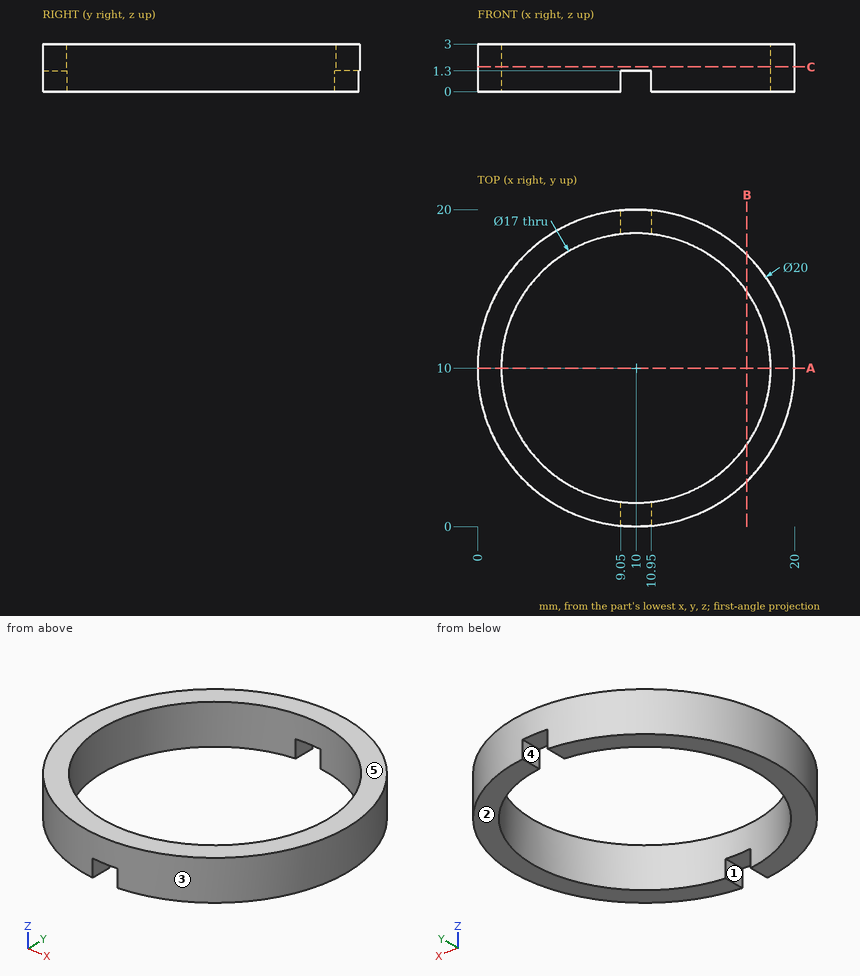
Part print with two shaded views. Sizes in mm from the minimum x, y, z corner. A direction names the side the tool comes from. Coordinates: 2 decimals unless noted, no trailing zeros. Order: outer loops, then holes, each group sorted by start corner. A loop starts at its lowest first (then second) coordinate and runs counter-clockwise, first axis right, second up. Notation, with made-up numbers: (69, 45) - (106, 45) arc R34 ccw to (106, 81) - close; hole circle Ø1 at (87.25, -31). An arc over 180 degrees is marked (long way). Answer in a Markdown table with one row per item.
1. Drill centre lines: L1, parallel to X at y = 10, z = 2; L2, parallel to X at y = 2.5, z = 2.85. Where is each one in solid material? Low to high. Write a range as from..to.
Answer:
| item | result |
|---|---|
| L1 | 0..1.5, 18.5..20 |
| L2 | 3.39..6, 14..16.61 |
2. Slice it at A-A, the plane y = 10. List the corners of the cut face in (x, z), then the cut area to 3 significant figures.
Answer:
| item | result |
|---|---|
| outline | (0, 0) - (1.5, 0) - (1.5, 3) - (0, 3) - close; (18.5, 0) - (20, 0) - (20, 3) - (18.5, 3) - close |
| area | 9.00 mm² |
3. Pull direction X, two halves, no side cores. Call the marked faces 3, 4 and 5: +X half, -X half, draft (parallel to the pull), parting line (faces both ways), or undercut.
Answer:
| item | result |
|---|---|
| face 3 | parting line |
| face 4 | undercut |
| face 5 | draft |
4. Slice it at B-B, the plane x = 17. List the corners of the cut face in (y, z).
Answer:
| item | result |
|---|---|
| outline | (2.86, 0) - (5.18, 0) - (5.18, 3) - (2.86, 3) - close; (14.82, 0) - (17.14, 0) - (17.14, 3) - (14.82, 3) - close |
5. 3-axis set-ups, long thin cutter, end or side, ignore diameter. For the marked faces 1 and 2: which of +Z, -Z, +X, -X, +Y, -Y reach the whole face in a straight line?
Answer:
| item | result |
|---|---|
| face 1 | -Z, +Y, -Y |
| face 2 | -Z, +X, -X, +Y, -Y |
6. Flat gauge pins, fed straight in: P1, Ø0.5, axis at x = 9.5, y = 19.5, coming from the -Z side; P2, Ø1.4, axis at y = 1, z = 1, coming from the -X side; P3, Ø1, axis at y = 1, z = 0.5, coming from the +X side. Where does each tip first touch, or does it go through?
Answer:
| item | result |
|---|---|
| P1 | z = 1.3 |
| P2 | x = 4.42 |
| P3 | x = 15.27 |
7. Slice it at C-C, the plane z = 1.55. List the corners of the cut face in (x, y).
Answer:
| item | result |
|---|---|
| outline | circle Ø20 at (10, 10); hole circle Ø17 at (10, 10) |
